Read the model definition and answer for the solid it produces. Units are mm, in the model's axes. Face numbers are marked on the shaded views. A direction names the side the tool comes from. Coordinates: 2 decimals unless noted, no trailing zeros. Order: outer loops, then holes, each group sorted by start corner. A loop starts at its lowest first (then second) coordinate and runs counter-clockwise, first axis right, second up. Notation, with made-up numbers: M -20,48.5 L 3,48.5 A14 ccw 3,60.5 Z; hole C 82,50.25 d2. An arc over 180 degrees is marked long. Write each question's results on one line, items separated by ' | '.
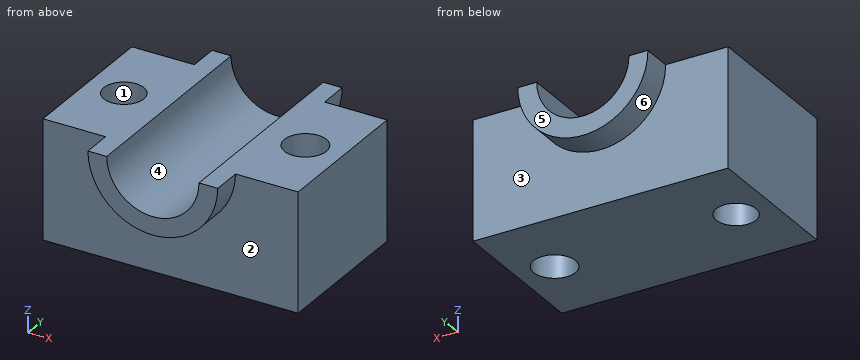
```python
from build123d import *

# Parameters (mm, degrees)
F0_W      = 108.991236
F0_H      = 63.794724
F1_DEPTH  = 50.8
F4_DEPTH  = 89.916
F5_DEPTH  = 12.7
F7_DEPTH  = 12.7
F8_R      = 8.535678
F9_DEPTH  = 76.708
F10_R     = 8.962055
F11_DEPTH = 88.392


with BuildPart() as f1:
    # F0 (on Top) → F1 (new body)
    with BuildSketch(Plane.XY):
        Rectangle(F0_W, F0_H)
    extrude(amount=F1_DEPTH)

    # F2 (on face) → F4 (cut)
    with BuildSketch(Plane.XZ.offset(31.897362)):
        with BuildLine():
            Line((19.697172, 50.8), (-19.697172, 50.8))
            ThreePointArc((-19.697172, 50.8), (0, 31.102828), (19.697172, 50.8))
        make_face()
    extrude(amount=-F4_DEPTH, mode=Mode.SUBTRACT)

    # F3 (on face) → F5 (join)
    with BuildSketch(Plane.XZ.offset(31.897362)):
        with BuildLine():
            Line((-19.697172, 50.8), (-27.762748, 50.8))
            ThreePointArc((-27.762748, 50.8), (0, 23.38646), (27.762748, 50.8))
            Line((27.762748, 50.8), (19.697172, 50.8))
            ThreePointArc((19.697172, 50.8), (0, 31.102828), (-19.697172, 50.8))
        make_face()
    extrude(amount=F5_DEPTH)

    # F6 (on face) → F7 (join)
    with BuildSketch(Plane(origin=(0, 31.897362, 0), x_dir=(-1, 0, 0), z_dir=(0, 1, 0))):
        with BuildLine():
            ThreePointArc((-27.800228, 50.8), (0, 22.999772), (27.800228, 50.8))
            Line((27.800228, 50.8), (19.697172, 50.8))
            ThreePointArc((19.697172, 50.8), (0, 31.102828), (-19.697172, 50.8))
            Line((-19.697172, 50.8), (-27.800228, 50.8))
        make_face()
    extrude(amount=F7_DEPTH)

    # F8 (on face) → F9 (cut)
    with BuildSketch(Plane.XY.offset(50.8)):
        with Locations((-38.936164, 0)):
            Circle(F8_R)
    extrude(amount=-F9_DEPTH, mode=Mode.SUBTRACT)

    # F10 (on face) → F11 (cut)
    with BuildSketch(Plane.XY.offset(50.8)):
        with Locations((38.630784, 0)):
            Circle(F10_R)
    extrude(amount=-F11_DEPTH, mode=Mode.SUBTRACT)


solid = f1.part
```
(1) The part is cut by section C-C, the plane z = 18. Write down the section's boundary in (x, y).
Conclusion:
outline: M -54.5,-31.9 L 54.5,-31.9 L 54.5,31.9 L -54.5,31.9 Z; hole C -38.94,0 d17.07; hole C 38.63,0 d17.92
(2) For the marked faces 5 and 6, determine the directions among +Z, -Z, +X, -X, +Y, -Y from which every point of the face is accessible in a straight line to the end or side of a thin tool.
Conclusion:
face 5: +Z, -Z, +X, -X, +Y | face 6: -Z, +Y
(3) The part is cut by section A-A, the plane z = 40.5. Write down the section's boundary in (x, y).
Conclusion:
outline: M -54.5,-31.9 L -25.64,-31.9 L -25.64,-44.6 L -16.79,-44.6 L -16.79,44.6 L -25.82,44.6 L -25.82,31.9 L -54.5,31.9 Z; M 16.79,-44.6 L 25.64,-44.6 L 25.64,-31.9 L 54.5,-31.9 L 54.5,31.9 L 25.82,31.9 L 25.82,44.6 L 16.79,44.6 Z; hole C -38.94,0 d17.07; hole C 38.63,0 d17.92
(4) The part is cut by section D-D, the plane x = 0. Write down the section's boundary in (y, z).
Conclusion:
outline: M -44.6,23.39 L -31.9,23.39 L -31.9,0 L 31.9,0 L 31.9,23 L 44.6,23 L 44.6,31.1 L -44.6,31.1 Z
(5) The part is cut by section B-B, the plane y = 0. Write down the section's boundary in (x, z).
Conclusion:
outline: M -54.5,0 L -47.47,0 L -47.47,50.8 L -54.5,50.8 Z; M -30.4,0 L 29.67,0 L 29.67,50.8 L 19.7,50.8 A19.7 cw -19.7,50.8 L -30.4,50.8 Z; M 47.59,0 L 54.5,0 L 54.5,50.8 L 47.59,50.8 Z
(6) The mould has two halves that part along Y. Classify the marked faces 1, 2, 3 and 4: pulls with the +Y half, pulls with the -Y half, needs draft (parallel to the pull), parting line crosses it, or undercut.
Conclusion:
face 1: undercut | face 2: pulls with the -Y half | face 3: pulls with the +Y half | face 4: needs draft
(7) Straight lines are drawn through the part: line 1 (X direction, y = -7, z = 12); line 2 (X direction, y = 1.5, z = 36.5); line 3 (X direction, y = 30, z = 43). For each, find the intervals that lie inside material, in ascending order.
Conclusion:
line 1: -54.5 to -43.82, -34.05 to 33.03, 44.23 to 54.5 | line 2: -54.5 to -47.34, -30.53 to -13.55, 13.55 to 29.8, 47.47 to 54.5 | line 3: -54.5 to -18.09, 18.09 to 54.5
